Check sheet for the modelled part. Datum: model origin and axes. Units: mm. Round coordinates to 2 decimals unless told otherwise and drop trailing zeros. Loops run counter-clockwise (first coordinate to the right, second up) from the corner with the lowest first, then second, coordinate; pieces in that order, holes last. Notation, with made-up numbers: (31.5, -22) -> (49.5, -22) arc R20 cw to (49.5, 17) -> close; hole circle Ø2 at (15.25, 8). An arc over 180 degrees is marked (long way). Use one line per item in the form item = value. Start each with the question number.
(1) Material ranges on probe 1 along X at (y, z) = (1.8, -30.85); probe 2 along Z at (x, y) = (43, 2.85); probe 3 along Z at (x, y) = (92, 1.7), recorded low to high. Write a range as [from, to].
(2) Sectioned sample at B-B (x = 60). Record the cut outline in (y, z).
(3) Sectioned sample at C-C (y = 1.9). Record the cut outline in (x, z), and give its area (3 significant figures).
(4) Go/stop test with a flat-tipped pin: pin 1 (4 mm diameter, centred on x = 12, z = -30.85, fed in from +Y). Record where the tip stops, or that it passes through.
(5) Sectioned sample at A-A (z = -17.8). Record the cut outline in (x, y).
(6) Sectioned sample at D-D (x = 12). Record the cut outline in (y, z), and give its area (3 significant figures).
from build123d import *

# Parameters (mm, degrees)
SKETCH_1_W          = 120
SKETCH_1_H          = 35.6
EXTRUDE_1_DEPTH     = 3
SKETCH_2_R          = 1.55
CUT_EXTRUDE_1_DEPTH = 3


with BuildPart() as part:
    # 草图1 → 凸台-拉伸1 (new body)
    with BuildSketch(Plane(origin=(0, 0, 0), x_dir=(1, 0, 0), z_dir=(0, 1, 0))):
        with Locations((60, 17.8)):
            Rectangle(SKETCH_1_W, SKETCH_1_H)
        with BuildLine():
            Line((30, 25.8), (90, 25.8))
            ThreePointArc((90, 25.8), (98, 17.8), (90, 9.8))
            Line((90, 9.8), (30, 9.8))
            ThreePointArc((30, 9.8), (22, 17.8), (30, 25.8))
        make_face(mode=Mode.SUBTRACT)
    extrude(amount=EXTRUDE_1_DEPTH)

    # 草图2 → 切除-拉伸1 (cut)
    with BuildSketch(Plane.XZ):
        with Locations((138, -4.75)):
            Circle(SKETCH_2_R)
        with Locations((138, -30.85)):
            Circle(SKETCH_2_R)
        with Locations(Location((12, -30.85, 0), (0, 0, 270))):
            Circle(SKETCH_2_R)
        with Locations(Location((12, -4.75, 0), (0, 0, 270))):
            Circle(SKETCH_2_R)
    extrude(amount=-CUT_EXTRUDE_1_DEPTH, mode=Mode.SUBTRACT)


solid = part.part
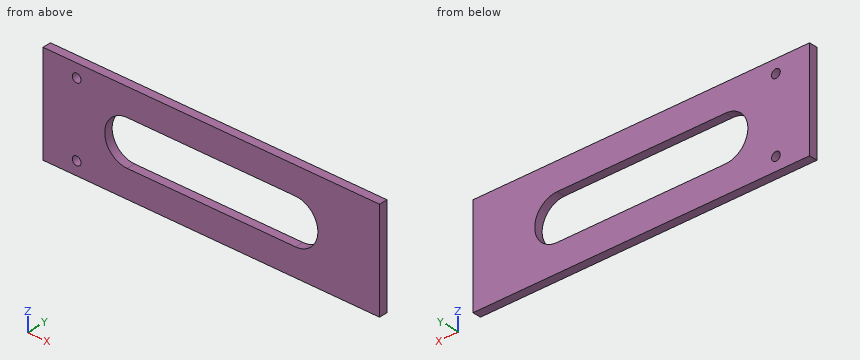
Checks:
q1.probe_1 = [0, 10.45], [13.55, 120]
q1.probe_2 = [-35.6, -25.8], [-9.8, 0]
q1.probe_3 = [-35.6, -25.55], [-10.05, 0]
q2.outline = (0, -35.6) -> (3, -35.6) -> (3, -25.8) -> (0, -25.8) -> close; (0, -9.8) -> (3, -9.8) -> (3, 0) -> (0, 0) -> close
q3.outline = (0, -35.6) -> (120, -35.6) -> (120, 0) -> (0, 0) -> close; hole circle Ø3.1 at (12, -30.85); hole circle Ø3.1 at (12, -4.75); hole (30, -25.8) -> (90, -25.8) arc R8 ccw to (90, -9.8) -> (30, -9.8) arc R8 ccw to start
q3.area = 3,100 mm2
q4.pin_1 = 3
q5.outline = (0, 0) -> (22, 0) -> (22, 3) -> (0, 3) -> close; (98, 0) -> (120, 0) -> (120, 3) -> (98, 3) -> close
q6.outline = (0, -35.6) -> (3, -35.6) -> (3, -32.4) -> (0, -32.4) -> close; (0, -29.3) -> (3, -29.3) -> (3, -6.3) -> (0, -6.3) -> close; (0, -3.2) -> (3, -3.2) -> (3, 0) -> (0, 0) -> close
q6.area = 88.2 mm2
